```python
from build123d import *

# Parameters (mm, degrees)
EXTRUSION1_DEPTH      = 20.2
EXTRUSION2_DEPTH      = 8.7
EXTRUSION3_DEPTH      = 11.5
EXTRUSION5_DEPTH      = 85.851864404
ESQUISSE7_R           = 5.5
EXTRUSION7_DEPTH      = 85.851864404
CHANFREIN1_SIZE       = 3
ESQUISSE11_W          = 6
ESQUISSE11_H          = 3.5
EXTRUSION10_DEPTH     = 2
ESQUISSE12_W          = 6
ESQUISSE12_H          = 22.2
EXTRUSION11_DEPTH     = 11.7
EXTRUSION12_START     = -6
EXTRUSION12_DEPTH     = 6
D_GAGEMENT_M61_D      = 6.6
D_GAGEMENT_M61_DEPTH  = 10
TROU_TARAUD_M62_D     = 5
ESQUISSE21_R          = 8
EXTRUSION13_DEPTH     = 97.102649527
ESQUISSE22_R          = 3.25
EXTRUSION14_DEPTH     = 74.818126201
TROU_TARAUD_M31_D     = 2.5
TROU_TARAUD_M31_DEPTH = 4.5
TROU_TARAUD_M31_TIP   = 0.751075774
TROU_TARAUD_M32_D     = 2.5
TROU_TARAUD_M32_DEPTH = 7.5
TROU_TARAUD_M32_TIP   = 0.751075774


with BuildPart() as part:
    # Esquisse1 → Extrusion1 (new body)
    with BuildSketch(Plane.XY):
        Polygon((-23.713097305, 25.832589029), (-23.713097305, -4.667410971), (14.886902695, -4.667410971), (14.886902695, -1.167410971), (-7.113097305, -1.167410971), (-7.113097305, 21.632589029), (-7.113097305, 25.832589029), (-29.411236045, 41.445913863), (-29.411236045, 53.045913863), (-49.463257995, 55.486490788), (-60.934786722, 39.103449903), (-51.4215104, 28.832248725), (-42.076114027, 27.820534025), align=None)
    extrude(amount=EXTRUSION1_DEPTH)

    # Esquisse2 → Extrusion2 (cut)
    with BuildSketch(Plane(origin=(0, 0, 0), x_dir=(-1, 0, 0), z_dir=(0, 0, -1))):
        Polygon((49.463257995, 55.486490788), (29.411236045, 41.445913863), (29.411236045, 53.045913863), align=None)
    extrude(amount=-EXTRUSION2_DEPTH, mode=Mode.SUBTRACT)

    # Esquisse3 → Extrusion3 (cut)
    with BuildSketch(Plane.XY.offset(20.2)):
        Polygon((-29.411236045, 41.445913863), (-35.397890495, 36.351131961), (-51.4215104, 28.832248725), (-23.713097305, 25.832589029), (-23.713097305, 21.632589029), (-7.113097305, 21.632589029), (-7.113097305, 25.832589029), align=None)
    extrude(amount=-EXTRUSION3_DEPTH, mode=Mode.SUBTRACT)

    # Esquisse5 → Extrusion5 (cut, through all)
    with BuildSketch(Plane.XY.offset(20.2)):
        Polygon((-56.059387013, 46.066242279), (-55.199022358, 47.294970345), (-48.383798942, 42.522899535), (-49.244163597, 41.294171468), align=None)
    extrude(amount=-EXTRUSION5_DEPTH, mode=Mode.SUBTRACT)

    # Esquisse7 → Extrusion7 (cut, through all)
    with BuildSketch(Plane(origin=(0, 0, 0), x_dir=(-1, 0, 0), z_dir=(0, 0, -1))):
        with Locations((44.350730044, 38.783333349)):
            Circle(ESQUISSE7_R)
    extrude(amount=-EXTRUSION7_DEPTH, mode=Mode.SUBTRACT)

    # Chanfrein1
    chanfrein1_edges = [part.edges().sort_by_distance(p)[0] for p in [
        (-15.413097305, 21.632589029, 20.2),
    ]]
    chamfer(chanfrein1_edges, length=CHANFREIN1_SIZE)

    # Esquisse11 → Extrusion10 (add)
    with BuildSketch(Plane(origin=(0, 0, 0), x_dir=(-1, 0, 0), z_dir=(0, 0, -1))):
        with Locations((-11.886902695, -2.917410971)):
            Rectangle(ESQUISSE11_W, ESQUISSE11_H)
    extrude(amount=EXTRUSION10_DEPTH)

    # Esquisse12 → Extrusion11 (add)
    with BuildSketch(Plane(origin=(0, -1.167410971, 0), x_dir=(-1, 0, 0), z_dir=(0, 1, 0))):
        with Locations((-11.886902695, 9.1)):
            Rectangle(ESQUISSE12_W, ESQUISSE12_H)
    extrude(amount=EXTRUSION11_DEPTH)

    # Esquisse13 → Extrusion12 (add)
    with BuildSketch(Plane(origin=(14.886902695, 0, 0), x_dir=(0, 0, -1), z_dir=(1, 0, 0)).offset(EXTRUSION12_START)):
        with BuildLine():
            Line((-20.2, 10.532589029), (2, 10.532589029))
            ThreePointArc((2, 10.532589029), (-9.1, 21.632589029), (-20.2, 10.532589029))
        make_face()
    extrude(amount=EXTRUSION12_DEPTH)

    # Dégagement M61
    with Locations(Plane(origin=(-45.470336254, 52.690616886, 4.293910537), x_dir=(0.819152044289, -0.573576436351, 0), z_dir=(0.573576436351, 0.819152044289, 0))):
        with Locations((1e-09, 0)):
            Hole(D_GAGEMENT_M61_D / 2, depth=D_GAGEMENT_M61_DEPTH)

    # Trou taraudé M62 (through all)
    with Locations(Plane(origin=(-52.066839949, 43.270630728, 4.294), x_dir=(0.819152044289, -0.573576436351, 0), z_dir=(0.573576436351, 0.819152044289, 0))):
        with Locations((0, 0)):
            Hole(TROU_TARAUD_M62_D / 2)

    # Esquisse21 → Extrusion13 (cut, through all)
    with BuildSketch(Plane(origin=(14.886902695, 0, 0), x_dir=(0, 0, -1), z_dir=(1, 0, 0))):
        with Locations((-9.1, 10.632589029)):
            Circle(ESQUISSE21_R)
    extrude(amount=-EXTRUSION13_DEPTH, mode=Mode.SUBTRACT)

    # Esquisse22 → Extrusion14 (cut, through all)
    with BuildSketch(Plane(origin=(-29.411236045, 0, 0), x_dir=(0, 0, -1), z_dir=(1, 0, 0))):
        with Locations(Location((-15.95, 47.545913863, 0), (0, 0, 90))):
            Circle(ESQUISSE22_R)
    extrude(amount=-EXTRUSION14_DEPTH, mode=Mode.SUBTRACT)

    # Trou taraudé M31
    with Locations(Plane(origin=(5.932756634, 48.744116607, 0), x_dir=(-0.992674353944791, 0.1208206398770179, 0), z_dir=(0.12082063987701788, 0.9926743539447909, 0))):
        with Locations((43.104820996, 15.95)):
            Hole(TROU_TARAUD_M31_D / 2, depth=TROU_TARAUD_M31_DEPTH)
            with Locations((0, 0, -(TROU_TARAUD_M31_DEPTH + TROU_TARAUD_M31_TIP / 2))):  # 118° drill point
                Cone(0, TROU_TARAUD_M31_D / 2, TROU_TARAUD_M31_TIP, mode=Mode.SUBTRACT)

    # Trou taraudé M32
    with Locations(Plane(origin=(14.886902695, 0.132589029, 17.7), x_dir=(0, 0, 1), z_dir=(1, 0, 0))):
        with Locations((0, 0)):
            Hole(TROU_TARAUD_M32_D / 2, depth=TROU_TARAUD_M32_DEPTH)
            with Locations((0, 0, -(TROU_TARAUD_M32_DEPTH + TROU_TARAUD_M32_TIP / 2))):  # 118° drill point
                Cone(0, TROU_TARAUD_M32_D / 2, TROU_TARAUD_M32_TIP, mode=Mode.SUBTRACT)


solid = part.part
```
Geometry: final body of the model. Coordinates: model frame, mm. A direction names the side the tool comes from. Give positions to 0.01 mm unless a question says otherwise; leave off trailing zeros. Loops run counter-clockwise (first coordinate to the right, second up) from the corner with the lowest first, then second, coordinate; pieces in that order, holes last. Notation, with made-up numbers: (68.5, 39) -> (121.5, 39) arc R16 cw to (121.5, 59) -> close; hole circle Ø8 at (81, -33). An arc over 180 degrees is marked (long way). Use one line per item in the form item = value.
Item 1: Section query A-A on y = 6. Output: boundary loops of the cut face in (x, z), and give its area (3 significant figures).
A:
outline = (-23.71, 0) -> (-7.11, 0) -> (-7.11, 2.58) -> (-23.71, 2.58) -> close; (-23.71, 15.62) -> (-7.11, 15.62) -> (-7.11, 20.2) -> (-23.71, 20.2) -> close; (8.89, -2) -> (14.89, -2) -> (14.89, 2.58) -> (8.89, 2.58) -> close; (8.89, 15.62) -> (14.89, 15.62) -> (14.89, 20.2) -> (8.89, 20.2) -> close
area = 174 mm^2
Item 2: Line query: probe 1 along X at (y, z) = (1, 8.5); probe 2 along Y at (x, z) = (-15.5, 9.1); probe 3 along Y at (x, z) = (11.05, 17.7). Output: solid intervals per line, ascending.
A:
probe_1 = -23.71 to -7.11, 8.89 to 14.89
probe_2 = -4.67 to 2.63, 18.63 to 21.63
probe_3 = -4.67 to -1.12, 1.38 to 17.55
Item 3: Section query B-B on z = 3. Give the number of separate pieces and of enclosed holes in the cut face, and give its area (3 significant figures).
A:
separate_pieces = 5
enclosed_holes = 0
area = 1,020 mm^2
Item 4: Access query for faces 1 (the face through (-23.713, 4, 14)), 2 (the face through (-52.29, 51.45, 9.96)), 3 (the face through (-43.298, 32.644, 14.53)), 4 (the face through (-51.839, 44.942, 10.241)). Directions: +Z, -Z, +X, -X, +Y, -Y. A direction counts if a zero-diameter tool reaches every point of the face in a straight line with its end or side. Return the directions, or none.
A:
face_1 = +Z, -Z, -X, -Y
face_2 = +Z, -Z, -X, +Y
face_3 = +Z, +X, -Y
face_4 = +Z, -Z
Item 5: Pin query (flat end, axial travel): P1, Ø5, axis at x = -42.5, z = 10, coming from the +Y side; P2, Ø9, axis at y = 46, z = 14.5, coming from the +X side; P3, Ø11, axis at x = -39.5, y = 47.5, coming from the -Z side. Return the tip coordinate at first contact, or that it passes through.
A:
P1 = 54.94
P2 = -29.41
P3 = 0
Item 6: Section query D-D on y = 24. Output: boundary loops of the cut face in (x, z).
A:
outline = (-23.71, 0) -> (-7.11, 0) -> (-7.11, 8.7) -> (-23.71, 8.7) -> close
Item 7: Section query C-C on x = -34. Output: boundary loops of the cut face in (y, z), and give its area (3 significant figures).
A:
outline = (26.95, 0) -> (44.66, 0) -> (44.66, 8.7) -> (53.6, 8.7) -> (53.6, 20.2) -> (37.54, 20.2) -> (37.54, 8.7) -> (26.95, 8.7) -> close; hole circle Ø6.5 at (47.55, 15.95)
area = 306 mm^2
Item 8: Draft query along Z for faces 5 (the face through (-4, -4.667, 9)), 6 (the face through (-55.765, 44.296, 16)), 7 (the face through (-26, 28, 0)), 8 (the face through (-50.875, 50.286, 5.558)). Return one class per face: pulls with the +Z half, pulls with the -Z half, needs draft (parallel to the pull), parting line crosses it, or undercut.
A:
face_5 = needs draft
face_6 = undercut
face_7 = pulls with the -Z half
face_8 = undercut
